Model file for the job. Use its own axes, mm. Face numbers are marked on the shaded views. A direction names the side the tool comes from. Give positions to 0.01 mm unless a question says otherwise; leave off trailing zeros. Order: outer loops, then holes, each group sorted by start corner. A loop starts at its lowest first (then second) coordinate and runs counter-clockwise, first axis right, second up. Notation, with made-up numbers: (-28.5, 55.5) - (-16.5, 55.5) arc R22 ccw to (-16.5, 67.5) - close; hole circle Ø8 at (25.25, -22). An arc over 180 degrees is marked (long way). Return JSON: item names as keys, results as strings. Group by question number.
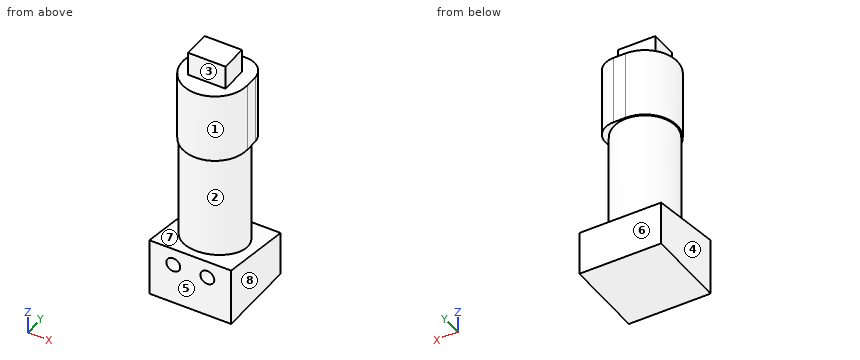
from build123d import *

# Parameters (mm, degrees)
CROQUIS1_W              = 24
CROQUIS1_H              = 17
SALIENTE_EXTRUIR1_DEPTH = 24
CORTAR_EXTRUIR1_DEPTH   = 24
CROQUIS4_R              = 9.125
SALIENTE_EXTRUIR3_DEPTH = 33.5
SALIENTE_EXTRUIR4_DEPTH = 20.5
CROQUIS6_W              = 11
CROQUIS6_H              = 8
SALIENTE_EXTRUIR5_DEPTH = 7
CROQUIS7_R              = 2.05
CORTAR_EXTRUIR2_DEPTH   = 6


with BuildPart() as part:
    # Croquis1 → Saliente-Extruir1 (new body)
    with BuildSketch(Plane(origin=(0, 0, 0), x_dir=(1, 0, 0), z_dir=(0, 1, 0))):
        Rectangle(CROQUIS1_W, CROQUIS1_H)
    extrude(amount=SALIENTE_EXTRUIR1_DEPTH)

    # Croquis2 → Cortar-Extruir1 (cut)
    with BuildSketch(Plane(origin=(12, 0, 0), x_dir=(0, 0, -1), z_dir=(1, 0, 0))):
        Polygon((-8.5, 0), (-4.500138715, 24), (-8.5, 24), align=None)
    extrude(amount=-CORTAR_EXTRUIR1_DEPTH, mode=Mode.SUBTRACT)

    # Croquis4 → Saliente-Extruir3 (add)
    with BuildSketch(Plane(origin=(0, 0, 4.500138715), x_dir=(1, 0, 0), z_dir=(0, 0, -1))):
        with Locations(Location((0, -12, 0), (0, 0, 180))):
            Circle(CROQUIS4_R)
    extrude(amount=-SALIENTE_EXTRUIR3_DEPTH)

    # Croquis5 → Saliente-Extruir4 (add)
    with BuildSketch(Plane.XY.offset(38.000138715)):
        with BuildLine():
            Line((0, 21.5), (3.522837546, 21.5))
            ThreePointArc((3.522837546, 21.5), (7.576354538, 19.923686246), (9.5, 16.023))
            Line((9.5, 16.023), (9.5, 12))
            ThreePointArc((9.5, 12), (-6.717514421, 5.282485579), (0, 21.5))
        make_face()
    extrude(amount=SALIENTE_EXTRUIR4_DEPTH)

    # Croquis6 → Saliente-Extruir5 (add)
    with BuildSketch(Plane.XY.offset(58.500138715)):
        with Locations((0, 12)):
            Rectangle(CROQUIS6_W, CROQUIS6_H)
    extrude(amount=SALIENTE_EXTRUIR5_DEPTH)

    # Croquis7 → Cortar-Extruir2 (cut)
    with BuildSketch(Plane.XZ):
        with Locations(Location((-5, 3.5, 0), (0, 0, 270))):
            Circle(CROQUIS7_R)
        with Locations(Location((5, 3.5, 0), (0, 0, 270))):
            Circle(CROQUIS7_R)
    extrude(amount=-CORTAR_EXTRUIR2_DEPTH, mode=Mode.SUBTRACT)


solid = part.part
(1) Drop flat-ended pins along their axis: pin 1 Ø2 at (x, z) = (-5.5, 3) entering from -Y; pin 2 Ø8 at (y, z) = (11, 27.5) entering from -X (3 decimals); pin 3 Ø3.5 at (x, z) = (-1.5, 61.5) entering from +Y; pin 4 Ø6.5 at (x, z) = (-5, 3.5) entering from -Y. Give the stop position or say it passes through.
(2) Slice it at C-C (z = 52). Give the cut face in (x, y).
(3) Drill centre lines: L1, parallel to X at y = 3.95, z = 3.5; L2, parallel to Z at x = 0.25, y = 7.5; L3, parallel to Y at x = 4.5, z = 3.5. Where is each one in solid material? Low to high.
(4) 3-axis set-ups, long thin cutter, end or side, ignore diameter. For the marked faces 1, 2, 3 and 4: which of +Z, -Z, +X, -X, +Y, -Y reach the whole face in a straight line?
(5) Slice it at A-A (z = 3.5). Give the cut face in (x, y), and give its area (3 significant figures).
(6) Slice it at B-B (y = 6.75). Give the cut face in (x, z), and give its area (3 significant figures).
(7) Pull direction Y, two halves, no side cores. Call the marked faces 5, 6, 7 and 8: released by +Y, released by -Y, zero draft, split by the parting line, or undercut.
(8) Slice it at D-D (y = 11.25). Give the cut face in (x, z), and give its area (3 significant figures).
Result set:
{
 "1": {"pin 1": "stops at y = 6", "pin 2": "stops at x = -9.125", "pin 3": "stops at y = 16", "pin 4": "stops at y = 0"},
 "2": {"outline": "(0, 21.5) arc R9.5 ccw (long way) to (9.5, 12) - (9.5, 16.02) arc R6 ccw to (3.52, 21.5) - close"},
 "3": {"L1": "x = -12 to -7.05, -2.95 to 2.95, 7.05 to 12", "L2": "z = -8.5 to 58.5", "L3": "y = 6 to 24"},
 "4": {"face 1": "+Z", "face 2": "none", "face 3": "+Z, +X, -X, -Y", "face 4": "+Z, -Z, -X, +Y, -Y"},
 "5": {"outline": "(-12, 0) - (-7.05, 0) - (-7.05, 6) - (-2.95, 6) - (-2.95, 0) - (2.95, 0) - (2.95, 6) - (7.05, 6) - (7.05, 0) - (12, 0) - (12, 24) - (-12, 24) - close", "area": "527 mm²"},
 "6": {"outline": "(-12, -8.5) - (12, -8.5) - (12, 7.38) - (7.46, 7.38) - (7.46, 38) - (7.92, 38) - (7.92, 58.5) - (-7.92, 58.5) - (-7.92, 38) - (-7.46, 38) - (-7.46, 7.38) - (-12, 7.38) - close", "area": "1,160 mm²"},
 "7": {"face 5": "released by -Y", "face 6": "released by +Y", "face 7": "undercut", "face 8": "zero draft"},
 "8": {"outline": "(-12, -8.5) - (12, -8.5) - (12, 6.63) - (9.09, 6.63) - (9.09, 38) - (9.47, 38) - (9.47, 58.5) - (5.5, 58.5) - (5.5, 65.5) - (-5.5, 65.5) - (-5.5, 58.5) - (-9.47, 58.5) - (-9.47, 38) - (-9.09, 38) - (-9.09, 6.63) - (-12, 6.63) - close", "area": "1,400 mm²"}
}
